Geometry: final body of the model. Coordinates: model frame, mm. A direction names the side the tool comes from. Give positions to 0.01 mm unless a question says otherwise; leave off trailing zeros. Order: outer loops, then holes, each group sorted by start corner. A loop starts at its lowest first (then second) coordinate and runs counter-clockwise, first axis right, second up. Notation, with made-up numbers: (44.25, -31) -> (74.25, -31) arc R26 ccw to (74.25, -2) -> close; hole circle Ø6 at (87, 52.5). An arc over 180 degrees is marked (long way). Answer in a Markdown table with one row per item. Add a question column.
Q1. Cut plane A-A on x = -55. Return the cut outline in (y, z).
Q2. Line query: line 1 along Y through (x, z) = (-37, -39); line 2 along X through (y, z) = (34, -9); line 3 along X through (y, z) = (17.5, -10.5). Output: solid intervals per line, ascending. Write a range as from..to.
Q3. Pull-direction query (X, two-part tool) for faces 1 (the face through (-2, 1, -50)), 2 (the face through (96, -26, -35)); classes: +X half, -X half, draft (parallel to the pull), parting line (faces both ways), or undercut.
Q4. Cut plane B-B on y = -38. Return the cut outline in (x, z).
Q5. Cut plane D-D on y = 46. Return the cut outline in (x, z).
Q6. Contact query for a flat-ended pin moving along its axis: P1, Ø5, axis at x = 20, y = 2, coming from the +Z side. Output: stop coordinate, or through.
Q7. Set-up query: faces 3 (the face through (-49.3, 31, -27)), 4 (the face through (-60, -65.5, -42)), 5 (the face through (-2, -91.5, -25)). Return all of +Z, -Z, +X, -X, +Y, -Y with unobstructed straight access to the full face (end or side cutting, diameter ignored); none if empty.
Q8. Cut plane C-C on x = 101. Return the cut outline in (y, z).
from build123d import *

# Parameters (mm, degrees)
SKETCH_W        = 249
SKETCH_H        = 183
PAD_DEPTH       = 50
POCKET_DEPTH    = 35
POCKET001_DEPTH = 50
POCKET002_DEPTH = 45


with BuildPart() as part:
    # Sketch → Pad (new body)
    with BuildSketch(Plane.XY):
        Rectangle(SKETCH_W, SKETCH_H)
    extrude(amount=-PAD_DEPTH)

    # Sketch001 → Pocket (cut)
    with BuildSketch(Plane.XY):
        with BuildLine():
            Line((-111, 26.5), (-8, 26.5))
            ThreePointArc((-6, 24.5), (-6.585786, 25.914214), (-8, 26.5))
            Line((-6, 24.5), (-6, -78.5))
            ThreePointArc((-8, -80.5), (-6.585786, -79.914214), (-6, -78.5))
            Line((-8, -80.5), (-111, -80.5))
            ThreePointArc((-113, -78.5), (-112.414214, -79.914214), (-111, -80.5))
            Line((-113, -78.5), (-113, 24.5))
            ThreePointArc((-111, 26.5), (-112.414214, 25.914214), (-113, 24.5))
        make_face()
        with BuildLine():
            Line((8, 26.5), (111, 26.5))
            ThreePointArc((113, 24.5), (112.414214, 25.914214), (111, 26.5))
            Line((113, 24.5), (113, -78.5))
            ThreePointArc((111, -80.5), (112.414214, -79.914214), (113, -78.5))
            Line((111, -80.5), (8, -80.5))
            ThreePointArc((6, -78.5), (6.585786, -79.914214), (8, -80.5))
            Line((6, -78.5), (6, 24.5))
            ThreePointArc((8, 26.5), (6.585786, 25.914214), (6, 24.5))
        make_face()
    extrude(amount=-POCKET_DEPTH, mode=Mode.SUBTRACT)

    # Sketch002 → Pocket001 (cut)
    with BuildSketch(Plane.XY):
        Polygon((-82.8, 4.5), (-89.3, 4.5), (-89.3, -58.5), (-82.8, -58.5), (-82.8, -65.5), (-35.8, -65.5), (-35.8, -58.5), (-29.3, -58.5), (-29.3, 4.5), (-35.8, 4.5), (-35.8, 11.5), (-82.8, 11.5), align=None)
        Polygon((35.8, 4.5), (29.3, 4.5), (29.3, -58.5), (35.8, -58.5), (35.8, -65.5), (82.8, -65.5), (82.8, -58.5), (89.3, -58.5), (89.3, 4.5), (82.8, 4.5), (82.8, 11.5), (35.8, 11.5), align=None)
    extrude(amount=-POCKET001_DEPTH, mode=Mode.SUBTRACT)

    # Sketch003 → Pocket002 (cut)
    with BuildSketch(Plane.XY):
        with BuildLine():
            ThreePointArc((-110.6, 80.3), (-112.014214, 79.714214), (-112.6, 78.3))
            Line((-112.6, 40.3), (-112.6, 78.3))
            ThreePointArc((-112.6, 40.3), (-112.014214, 38.885786), (-110.6, 38.3))
            Line((-110.6, 38.3), (-69.3, 38.3))
            Line((-69.3, 38.3), (-69.3, 4.5))
            Line((-69.3, 4.5), (-89.3, 4.5))
            Line((-89.3, 4.5), (-89.3, -58.5))
            Line((-89.3, -58.5), (-82.8, -58.5))
            Line((-82.8, -58.5), (-82.8, -65.5))
            Line((-82.8, -65.5), (-35.8, -65.5))
            Line((-35.8, -65.5), (-35.8, -58.5))
            Line((-35.8, -58.5), (-29.3, -58.5))
            Line((-29.3, -58.5), (-29.3, 4.5))
            Line((-29.3, 4.5), (-49.3, 4.5))
            Line((-49.3, 4.5), (-49.3, 38.3))
            Line((-49.3, 38.3), (49.3, 38.3))
            Line((49.3, 38.3), (49.3, 4.5))
            Line((49.3, 4.5), (29.3, 4.5))
            Line((29.3, 4.5), (29.3, -58.5))
            Line((29.3, -58.5), (35.8, -58.5))
            Line((35.8, -58.5), (35.8, -65.5))
            Line((35.8, -65.5), (82.8, -65.5))
            Line((82.8, -65.5), (82.8, -58.5))
            Line((82.8, -58.5), (89.3, -58.5))
            Line((89.3, -58.5), (89.3, 4.5))
            Line((89.3, 4.5), (69.3, 4.5))
            Line((69.3, 4.5), (69.3, 38.3))
            Line((69.3, 38.3), (110.599996, 38.3))
            ThreePointArc((110.599996, 38.3), (112.01421, 38.885786), (112.599996, 40.3))
            Line((112.599996, 78.3), (112.599996, 40.3))
            ThreePointArc((112.599996, 78.3), (112.01421, 79.714214), (110.599996, 80.3))
            Line((-110.6, 80.3), (110.599996, 80.3))
        make_face()
    extrude(amount=-POCKET002_DEPTH, mode=Mode.SUBTRACT)


solid = part.part
Completed:
| question | item | result |
|---|---|---|
| 1 | outline | (-91.5, -50) -> (-65.5, -50) -> (-65.5, -35) -> (-80.5, -35) -> (-80.5, 0) -> (-91.5, 0) -> close; (11.5, -50) -> (91.5, -50) -> (91.5, 0) -> (80.3, 0) -> (80.3, -45) -> (11.5, -45) -> close |
| 2 | line 1 | y = -91.5..-65.5, 11.5..38.3, 80.3..91.5 |
| 2 | line 2 | x = -124.5..-69.3, -49.3..49.3, 69.3..124.5 |
| 2 | line 3 | x = -124.5..-113, -6..6, 113..124.5 |
| 3 | face 1 | draft |
| 3 | face 2 | undercut |
| 4 | outline | (-124.5, -50) -> (-89.3, -50) -> (-89.3, -35) -> (-113, -35) -> (-113, 0) -> (-124.5, 0) -> close; (-29.3, -50) -> (29.3, -50) -> (29.3, -35) -> (6, -35) -> (6, 0) -> (-6, 0) -> (-6, -35) -> (-29.3, -35) -> close; (89.3, -50) -> (124.5, -50) -> (124.5, 0) -> (113, 0) -> (113, -35) -> (89.3, -35) -> close |
| 5 | outline | (-124.5, -50) -> (124.5, -50) -> (124.5, 0) -> (112.6, 0) -> (112.6, -45) -> (-112.6, -45) -> (-112.6, 0) -> (-124.5, 0) -> close |
| 6 | P1 | stops at z = -35 |
| 7 | face 3 | +Z |
| 7 | face 4 | +Z, -Z |
| 7 | face 5 | +Z, -Z, +X, -X, -Y |
| 8 | outline | (-91.5, -50) -> (91.5, -50) -> (91.5, 0) -> (80.3, 0) -> (80.3, -45) -> (38.3, -45) -> (38.3, 0) -> (26.5, 0) -> (26.5, -35) -> (-80.5, -35) -> (-80.5, 0) -> (-91.5, 0) -> close |
